Autodesk Fusion 360 part; units mm, degrees
sketch "Esquisse1" plane through (0, 0, 0) normal (0, 0, 1) x (1, 0, 0)
  circle A0 centre (0, 0) radius 5
  circle A1 centre (0, 0) radius 4.2
  dimension "d1" = 10
  dimension "d2" = 8.4
extrude "Extrusion1" add sketch "Esquisse1" along normal blind 49.9
chamfer "Chanfrein1" distance 0.2 angle 45 1 edges at (-4.6616, -1.8081, 49.9)
chamfer "Chanfrein2" distance 0.2 angle 45 1 edges at (-4.6616, -1.8081, 0)
Work out the finished part from the listing and answer in its coordinate system (mm). Round coordinates to 2 decimals unless told otherwise and drop trailing zeros. Loops run counter-clockwise (first coordinate to the right, second up) from the corner with the lowest first, then second, coordinate; pieces in that order, holes last. Notation, with made-up numbers: (31, 44.5) - (35, 44.5) arc R11 cw to (35, 50.5) - close; hole circle Ø9 at (83, 76). An arc over 180 degrees is marked (long way). Use one line per item in the form item = value. Start each with the question number.
(1) Find section A-A on y = 0. Determine the outline of the cut face in (x, z).
(2) Consider line 1 (Y direction, x = 0, z = 31); line 2 (Y direction, x = 1.75, z = 18.5); line 3 (X direction, y = 0.5, z = 8). Determine where each line is inside the solid, lowest interval first.
(3) Find section C-C on z = 47. Determine the outline of the cut face in (x, y), and give its area (3 significant figures).
(4) Flat-ended cylindrical pins translate along their axes: P1, Ø1, axis at y = -2, z = 14, coming from the -X side; P2, Ø4, axis at x = -4, z = 21, coming from the -Y side; P3, Ø2, axis at y = -3.5, z = 21, coming from the +X side. Find the tip coordinate at first contact, or state that the pin passes through.
(5) Determine the mould class of faces 1 (the face through (4.006, -1.262, 24.601)), 2 (the face through (-1.08, 4.88, 24.6)), 3 (the face through (2, -4, 0)) for opening direction Y: +Y half, -Y half, draft (parallel to the pull), parting line (faces both ways), or undercut.
Answer list:
q1.outline = (-5, 0.2) - (-4.8, 0) - (-4.2, 0) - (-4.2, 49.9) - (-4.8, 49.9) - (-5, 49.7) - close; (4.2, 0) - (4.8, 0) - (5, 0.2) - (5, 49.7) - (4.8, 49.9) - (4.2, 49.9) - close
q2.line_1 = -5 to -4.2, 4.2 to 5
q2.line_2 = -4.68 to -3.82, 3.82 to 4.68
q2.line_3 = -4.97 to -4.17, 4.17 to 4.97
q3.outline = circle Ø10 at (0, 0); hole circle Ø8.4 at (0, 0)
q3.area = 23.1 mm^2
q4.P1 = -4.77
q4.P2 = -4.58
q4.P3 = 4.33
q5.face_1 = undercut
q5.face_2 = parting line
q5.face_3 = draft
